from build123d import *

# Parameters (mm, degrees)
F0_W     = 31.75
F0_H     = 31.75
F0_R     = 2.38125
F1_DEPTH = 9.525
F2_DEPTH = 11.1125
F3_W     = 15.875
F3_H     = 15.875
F4_DEPTH = 12.7
F5_R     = 2.38125
F6_DEPTH = 50.8
F8_DEPTH = 50.8


with BuildPart() as f1:
    # F0 (on Top) → F1 (new body)
    with BuildSketch(Plane.XY):
        Rectangle(F0_W, F0_H)
        with Locations((-11.90625, -11.90625)):
            Circle(F0_R, mode=Mode.SUBTRACT)
        with Locations((-3.96875, -11.90625)):
            Circle(F0_R, mode=Mode.SUBTRACT)
        with Locations((-11.90625, -3.96875)):
            Circle(F0_R, mode=Mode.SUBTRACT)
        with Locations((-3.96875, -3.96875)):
            Circle(F0_R, mode=Mode.SUBTRACT)
        with Locations((3.96875, -11.90625)):
            Circle(F0_R, mode=Mode.SUBTRACT)
        with Locations((11.90625, -11.90625)):
            Circle(F0_R, mode=Mode.SUBTRACT)
        with Locations((3.96875, -3.96875)):
            Circle(F0_R, mode=Mode.SUBTRACT)
        with Locations((11.90625, -3.96875)):
            Circle(F0_R, mode=Mode.SUBTRACT)
        with Locations((-11.90625, 3.96875)):
            Circle(F0_R, mode=Mode.SUBTRACT)
        with Locations((-3.96875, 3.96875)):
            Circle(F0_R, mode=Mode.SUBTRACT)
        with Locations((-11.90625, 11.90625)):
            Circle(F0_R, mode=Mode.SUBTRACT)
        with Locations((-3.96875, 11.90625)):
            Circle(F0_R, mode=Mode.SUBTRACT)
        with Locations((3.96875, 3.96875)):
            Circle(F0_R, mode=Mode.SUBTRACT)
        with Locations((11.90625, 3.96875)):
            Circle(F0_R, mode=Mode.SUBTRACT)
        with Locations((3.96875, 11.90625)):
            Circle(F0_R, mode=Mode.SUBTRACT)
        with Locations((11.90625, 11.90625)):
            Circle(F0_R, mode=Mode.SUBTRACT)
    extrude(amount=F1_DEPTH)

    # F0 (on Top) → F2 (join)
    with BuildSketch(Plane.XY):
        with Locations((-11.90625, 11.90625)):
            Circle(F0_R)
        with Locations((-3.96875, 11.90625)):
            Circle(F0_R)
        with Locations((3.96875, 11.90625)):
            Circle(F0_R)
        with Locations((11.90625, 11.90625)):
            Circle(F0_R)
        with Locations((11.90625, 3.96875)):
            Circle(F0_R)
        with Locations((3.96875, 3.96875)):
            Circle(F0_R)
        with Locations((-3.96875, 3.96875)):
            Circle(F0_R)
        with Locations((-11.90625, 3.96875)):
            Circle(F0_R)
        with Locations((-11.90625, -3.96875)):
            Circle(F0_R)
        with Locations((-3.96875, -3.96875)):
            Circle(F0_R)
        with Locations((3.96875, -3.96875)):
            Circle(F0_R)
        with Locations((11.90625, -3.96875)):
            Circle(F0_R)
        with Locations((11.90625, -11.90625)):
            Circle(F0_R)
        with Locations((3.96875, -11.90625)):
            Circle(F0_R)
        with Locations((-3.96875, -11.90625)):
            Circle(F0_R)
        with Locations((-11.90625, -11.90625)):
            Circle(F0_R)
    extrude(amount=F2_DEPTH)

    # F3 (on face) → F4 (cut, symmetric)
    with BuildSketch(Plane.XY.offset(9.525)):
        Rectangle(F3_W, F3_H)
    extrude(amount=F4_DEPTH, both=True, mode=Mode.SUBTRACT)

    # F5 (on face) → F6 (cut)
    with BuildSketch(Plane.XZ.offset(15.875)):
        with Locations((7.9375, 5.55625)):
            Circle(F5_R)
        with Locations((0, 5.55625)):
            Circle(F5_R)
        with Locations((-7.9375, 5.55625)):
            Circle(F5_R)
    extrude(amount=-F6_DEPTH, mode=Mode.SUBTRACT)

    # F7 (on face) → F8 (cut)
    with BuildSketch(Plane(origin=(-15.875, 0, 0), x_dir=(0, -1, 0), z_dir=(-1, 0, 0))):
        with BuildLine():
            ThreePointArc((0, 3.175), (1.683798, 3.872452), (2.38125, 5.55625))
            ThreePointArc((2.38125, 5.55625), (-1.683798, 7.240048), (0, 3.175))
        make_face()
    extrude(amount=-F8_DEPTH, mode=Mode.SUBTRACT)


solid = f1.part
Design review of the part built by this model. Coordinates are the model's own, in mm. A direction names the side the tool comes from. Round coordinates to 2 decimals unless told otherwise and drop trailing zeros. Write each loop counter-clockwise with the first axis right and the second up, starting at its lowest first coordinate (ties: lowest second). Pieces come first, ordered by that corner, then holes. Notation, with made-up numbers: M 57.5,19.25 L 88.5,19.25 A15 ccw 88.5,36.25 Z; hole C 60.25,-20.75 d5. An arc over 180 degrees is marked long. One line per item, written item: value. Start each with the question number.
1. Draft analysis for pull direction X (two halves, no side actions). For faces 1 (the face through (10.151, 5.578, 10.308)), 2 (the face through (-15.875, 0, 3)), 3 (the face through (4, -12, 11.112)), state which applies: pulls with the +X half, pulls with the -X half, needs draft (parallel to the pull), parting line crosses it, or undercut.
2. Take a section at D-D on x = -8.5. State the section outline as (y, z) points (1 decimal), then the cut area to 3 significant figures.
3. Take a section at B-B on y = -4.5. State the section outline as (x, z) points (1 decimal), then the cut area to 3 significant figures.
4. Clearance check with flat-ended pins moving along their axes: P1, Ø6, axis at y = 0, z = 5.56, coming from the +X side (3 decimals); P2, Ø1, axis at x = 9, y = 1, coming from the +Z side (3 decimals). State where each tip first meets the part, or that it passes through.
5. For faces 4 (the face through (-7.938, 0, 2)), 5 (the face through (-13.66, 5.58, 10.31)), 6 (the face through (-0.31, 11.851, 7.917)), list the 3-axis set-ups (+Z, -Z, +X, -X, +Y, -Y) from which the entire face can be reached by the end or side of a thin tool; tool diameter is ignored.
6. Take a section at C-C on y = 2. State the section outline as (x, z) points (1 decimal).
7. Take a section at A-A on x = 0. State the section outline as (y, z) points (1 decimal).
8. To check wall thickness, follow probe 1 along Y at (x, z) = (-11.5, 10.5); probe 2 along X at (y, z) = (8.5, 6.5) (3 decimals); probe 3 along Y at (x, z) = (2.5, 8.75) (1 decimal). State the ranges of each line that lie inside material, in increasing order. Write a range as from..to.
Computed:
1. face 1: undercut
1. face 2: pulls with the -X half
1. face 3: needs draft
2. outline: M -15.9,0 L 15.9,0 L 15.9,3.2 L 0.6,3.2 A2.4 cw -0.6,3.2 L -15.9,3.2 Z; M -15.9,7.9 L -0.6,7.9 A2.4 cw 0.6,7.9 L 15.9,7.9 L 15.9,9.5 L -15.9,9.5 Z
2. area: 155 mm²
3. outline: M -15.9,0 L -7.9,0 L -7.9,3.2 A2.4 cw -7.9,7.9 L -7.9,9.5 L -9.6,9.5 L -9.6,11.1 L -14.2,11.1 L -14.2,9.5 L -15.9,9.5 Z; M 7.9,0 L 15.9,0 L 15.9,9.5 L 14.2,9.5 L 14.2,11.1 L 9.6,11.1 L 9.6,9.5 L 7.9,9.5 L 7.9,7.9 A2.4 cw 7.9,3.2 Z
3. area: 148 mm²
4. P1: stops at x = 15.875
4. P2: stops at z = 9.525
5. face 4: +Z, -Z
5. face 5: +Z
5. face 6: +Y, -Y
6. outline: M -15.9,0 L -7.9,0 L -7.9,3.2 A2.4 cw -9.9,4.3 L -15.9,4.3 Z; M -15.9,6.8 L -9.9,6.8 A2.4 cw -7.9,7.9 L -7.9,9.5 L -10.6,9.5 L -10.6,11.1 L -13.2,11.1 L -13.2,9.5 L -15.9,9.5 Z; M 7.9,0 L 15.9,0 L 15.9,4.3 L 9.9,4.3 A2.4 cw 7.9,3.2 Z; M 7.9,7.9 A2.4 cw 9.9,6.8 L 15.9,6.8 L 15.9,9.5 L 13.2,9.5 L 13.2,11.1 L 10.6,11.1 L 10.6,9.5 L 7.9,9.5 Z
7. outline: M -15.9,0 L -7.9,0 L -7.9,3.2 L -15.9,3.2 Z; M -15.9,7.9 L -7.9,7.9 L -7.9,9.5 L -15.9,9.5 Z; M 7.9,0 L 15.9,0 L 15.9,3.2 L 7.9,3.2 Z; M 7.9,7.9 L 15.9,7.9 L 15.9,9.5 L 7.9,9.5 Z
8. probe 1: y = -14.25..-9.56, -6.32..-1.62, 1.62..6.32, 9.56..14.25
8. probe 2: x = -15.875..-10.124, -5.751..-2.186, 2.186..5.751, 10.124..15.875
8. probe 3: y = -15.9..-7.9, 7.9..15.9
